from build123d import *

# Parameters (mm, degrees)
BOSS_EXTRUDE1_DEPTH                      = 17.5
SKETCH3_OUTSIDE_W                        = 131.318
SKETCH3_OUTSIDE_H                        = 122.036
SKETCH3_OUTSIDE_R                        = 30
CUT_EXTRUDE1_DEPTH                       = 17.5
CUT_EXTRUDE1_TAPER                       = 30
CUT_EXTRUDE1_OTHER_WAY_DEPTH             = 17.5
CUT_EXTRUDE1_OTHER_WAY_TAPER             = 30
CBORE_FOR_M30_HEX_HEAD_BOLT1_D           = 33
CBORE_FOR_M30_HEX_HEAD_BOLT1_CBORE_D     = 56.116
CBORE_FOR_M30_HEX_HEAD_BOLT1_CBORE_DEPTH = 18.7


with BuildPart() as part:
    # Sketch2 → Boss-Extrude1 (new, symmetric)
    with BuildSketch(Plane.XY):
        Polygon((34.641016151, 0), (17.320508076, 30), (-17.320508076, 30), (-34.641016151, 0), (-17.320508076, -30), (17.320508076, -30), align=None)
    extrude(amount=BOSS_EXTRUDE1_DEPTH, both=True)

    # Sketch3 outside → Cut-Extrude1 (cut)
    with BuildSketch(Plane.XY.offset(17.5)):
        Rectangle(SKETCH3_OUTSIDE_W, SKETCH3_OUTSIDE_H)
        Circle(SKETCH3_OUTSIDE_R, mode=Mode.SUBTRACT)
    extrude(amount=CUT_EXTRUDE1_DEPTH, taper=CUT_EXTRUDE1_TAPER, mode=Mode.SUBTRACT)

    # Sketch3 outside → Cut-Extrude1 other way (cut)
    with BuildSketch(Plane.XY.offset(17.5)):
        Rectangle(SKETCH3_OUTSIDE_W, SKETCH3_OUTSIDE_H)
        Circle(SKETCH3_OUTSIDE_R, mode=Mode.SUBTRACT)
    extrude(amount=-CUT_EXTRUDE1_OTHER_WAY_DEPTH, taper=CUT_EXTRUDE1_OTHER_WAY_TAPER, mode=Mode.SUBTRACT)

    # CBORE for M30 Hex Head Bolt1 (through all)
    with Locations(Plane.XY.offset(17.5)):
        with Locations((0, 0)):
            CounterBoreHole(CBORE_FOR_M30_HEX_HEAD_BOLT1_D / 2, CBORE_FOR_M30_HEX_HEAD_BOLT1_CBORE_D / 2, CBORE_FOR_M30_HEX_HEAD_BOLT1_CBORE_DEPTH)


solid = part.part
Verification items for the finished model (mm, model axes). A direction names the side the tool comes from. Give positions to 0.01 mm unless a question says otherwise; leave off trailing zeros. Loops run counter-clockwise (first coordinate to the right, second up) from the corner with the lowest first, then second, coordinate; pieces in that order, holes last. Notation, with made-up numbers: (-19.75, -19) - (13.25, -19) arc R28 cw to (13.25, 17) - close; hole circle Ø11 at (18.25, -28.5). An arc over 180 degrees is marked (long way). Write item = value, one per line. Start each with the question number.
Q1. Cross-section at A-A, the plane z = -15. Enter the section's corners in (x, y), and give its area (3 significant figures).
Q2. Thickness scan on line 1 (Y direction, x = 0, z = -8); line 2 (Z direction, x = 5.5, y = -17); line 3 (X direction, y = 21.5, z = 5). Record the ranges inside material, lowest first.
Q3. Depth check by flat-ended pin: P1, Ø10, axis at y = 7, z = -12, coming from the -X side; P2, Ø1, axis at y = 19.5, z = 5.5, coming from the +X side; P3, Ø12, axis at x = -16.5, y = -16.5, coming from the +Z side; P4, Ø5, axis at y = 20.5, z = 7.5, coming from the -X side. Enter the tip coordinate at first touch or a pass-through.
Q4. Mould release check, pull along X, two halves, no side actions. Record for faces 3 (the face through (26.1, 14.79, 0.25)), 4 (the face through (26.76, 8.43, 8.28)), 5 (the face through (-15.498, -26.996, 15.546)): released by +X, released by -X, zero draft, split by the parting line, or undercut.
Q5. Cross-section at B-B, the plane z = 6.5. Enter the section's corners in (x, y).
Q6. Tool access check on faces 1 (the face through (12, -12, -1.2)), 2 (the face through (15, 14, -17.5)). Record the directions out of +Z, -Z, +X, -X, +Y, -Y that give a thin tool (end or side, any length) a straight path to the whole face; none if there is none.
Answer key:
q1.outline = (-34.64, 0) - (-17.32, -30) - (17.32, -30) - (34.64, 0) - (17.32, 30) - (-17.32, 30) - close; hole circle Ø33 at (0, 0)
q1.area = 2,260 mm^2
q2.line_1 = -30 to -16.5, 16.5 to 30
q2.line_2 = -17.5 to -1.2
q2.line_3 = -22.23 to -18.03, 18.03 to 22.23
q3.P1 = -33.49
q3.P2 = 23.67
q3.P3 = 17.5
q3.P4 = -24.25
q4.face_3 = released by +X
q4.face_4 = undercut
q4.face_5 = released by -X
q5.outline = (-34.64, 0) - (-17.32, -30) - (17.32, -30) - (34.64, 0) - (17.32, 30) - (-17.32, 30) - close; hole circle Ø56.12 at (0, 0)
q6.face_1 = +Z
q6.face_2 = -Z, +X, -X, +Y, -Y
